```python
from build123d import *

# Parameters (mm, degrees)
SKETCH_1_W          = 20
SKETCH_1_H          = 20
SKETCH_1_W_2        = 16
SKETCH_1_H_2        = 16
EXTRUDE_1_DEPTH     = 560
SKETCH_3_R          = 2.2
CUT_EXTRUDE_2_DEPTH = 560
SKETCH_4_R          = 2.2
CUT_EXTRUDE_3_DEPTH = 560
SKETCH_5_W          = 35.553041162
SKETCH_5_H          = 54.410354854
CUT_EXTRUDE_4_DEPTH = 40
SKETCH_6_W          = 32.938502486
SKETCH_6_H          = 36.721798984
CUT_EXTRUDE_5_DEPTH = 40
SKETCH_8_R          = 1
CUT_EXTRUDE_7_DEPTH = 10
M4X0_7_1_D          = 3.3
M4X0_7_1_DEPTH      = 11.5
M4X0_7_1_TIP        = 0.991420021


with BuildPart() as part:
    # ｽｹｯﾁ1 → ﾎﾞｽ - 押し出し1 (new body)
    with BuildSketch(Plane.XY):
        Rectangle(SKETCH_1_W, SKETCH_1_H)
        Rectangle(SKETCH_1_W_2, SKETCH_1_H_2, mode=Mode.SUBTRACT)
    extrude(amount=EXTRUDE_1_DEPTH)

    # ｽｹｯﾁ3 → ｶｯﾄ - 押し出し2 (cut)
    with BuildSketch(Plane(origin=(10, 0, 0), x_dir=(0, 0, -1), z_dir=(1, 0, 0))):
        with Locations((-530, 0)):
            Circle(SKETCH_3_R)
        with Locations((-30, 0)):
            Circle(SKETCH_3_R)
    extrude(amount=-CUT_EXTRUDE_2_DEPTH, mode=Mode.SUBTRACT)

    # ｽｹｯﾁ4 → ｶｯﾄ - 押し出し3 (cut)
    with BuildSketch(Plane(origin=(0, 10, 0), x_dir=(1, 0, 0), z_dir=(0, 1, 0))):
        with Locations((0, -550)):
            Circle(SKETCH_4_R)
        with Locations((0, -10)):
            Circle(SKETCH_4_R)
    extrude(amount=-CUT_EXTRUDE_3_DEPTH, mode=Mode.SUBTRACT)

    # ｽｹｯﾁ5 → ｶｯﾄ - 押し出し4 (cut)
    with BuildSketch(Plane(origin=(0, 0, 0), x_dir=(-1, 0, 0), z_dir=(0, 0, -1))):
        Rectangle(SKETCH_5_W, SKETCH_5_H)
    extrude(amount=-CUT_EXTRUDE_4_DEPTH, mode=Mode.SUBTRACT)

    # ｽｹｯﾁ6 → ｶｯﾄ - 押し出し5 (cut)
    with BuildSketch(Plane.XY.offset(560)):
        Rectangle(SKETCH_6_W, SKETCH_6_H)
    extrude(amount=-CUT_EXTRUDE_5_DEPTH, mode=Mode.SUBTRACT)

    # ｽｹｯﾁ8 → ｶｯﾄ - 押し出し7 (cut)
    with BuildSketch(Plane(origin=(10, 0, 0), x_dir=(0, 0, -1), z_dir=(1, 0, 0))):
        with Locations((-50, 0)):
            Circle(SKETCH_8_R)
        with Locations((-70, 0)):
            Circle(SKETCH_8_R)
        with Locations((-490, 0)):
            Circle(SKETCH_8_R)
        with Locations((-510, 0)):
            Circle(SKETCH_8_R)
    extrude(amount=-CUT_EXTRUDE_7_DEPTH, mode=Mode.SUBTRACT)

    # M4x0.7 ねじ穴1
    with Locations(Plane(origin=(10, 0, 50), x_dir=(0, 0, 1), z_dir=(1, 0, 0))):
        with Locations((0, 0), (20, 0), (440, 0), (460, 0)):
            Hole(M4X0_7_1_D / 2, depth=M4X0_7_1_DEPTH)
            with Locations((0, 0, -(M4X0_7_1_DEPTH + M4X0_7_1_TIP / 2))):  # 118° drill point
                Cone(0, M4X0_7_1_D / 2, M4X0_7_1_TIP, mode=Mode.SUBTRACT)


solid = part.part
```
Source: CAD feature listing. Evaluate the final solid. Frame: model axes, mm. A direction names the side the tool comes from. Round coordinates to 2 decimals unless told otherwise and drop trailing zeros. Loops run counter-clockwise (first coordinate to the right, second up) from the corner with the lowest first, then second, coordinate; pieces in that order, holes last.
1. Section query B-B on z = 479.5. Output: boundary loops of the cut face in (x, y), and give its area (3 significant figures).
2. Contact query for a flat-ended pin moving along its axis: pin 1 (2 mm diameter, centred on y = 0, z = 70, fed in from +X). Output: stop coordinate, or through.
3. Section query A-A on x = 0.5. Output: boundary loops of the cut face in (y, z).
4. Mould query, pull axis Y, two halves, no side actions, for faces 1 (the flat face through (0, 10, 277)), 2 (the flat face through (10, 0, 277)), 3 (the flat face through (-8, 0, 277)), 4 (the flat face through (8, 0, 277)). Classes: released by +Y, released by -Y, zero draft, split by the parting line, or undercut.
5. Access query for faces 5 (the flat face through (0, -10, 277)), 6 (the flat face through (0, 8, 277)). Directions: +Z, -Z, +X, -X, +Y, -Y. A direction counts if a zero-diameter tool reaches every point of the face in a straight line with its end or side. Return the directions, or none.
6. Ray query, L1, parallel to Y at x = 8.65, z = 510; L2, parallel to X at y = -4.25, z = 369. Return the intervals inside material, ascending.
Answers below:
1. outline: (-10, -10) - (10, -10) - (10, 10) - (-10, 10) - close; hole (-8, -8) - (8, -8) - (8, 8) - (-8, 8) - close
1. area: 144 mm2
2. pin 1: stops at x = -8
3. outline: (-10, 40) - (-8, 40) - (-8, 520) - (-10, 520) - close; (8, 40) - (10, 40) - (10, 520) - (8, 520) - close
4. face 1: released by +Y
4. face 2: zero draft
4. face 3: undercut
4. face 4: undercut
5. face 5: +Z, -Z, +X, -X, -Y
5. face 6: +Z, -Z
6. L1: y = -10 to -1.65, 1.65 to 10
6. L2: x = -10 to -8, 8 to 10
